For this review, take the finished solid that the model builds, in its own axes (mm). Round coordinates to 2 decimals unless told otherwise and drop trailing zeros. Write each loop counter-clockwise with the first axis right and the second up, starting at its lowest first coordinate (ties: lowest second). Pieces come first, ordered by that corner, then holes. Notation, with made-up numbers: (-36, 29) -> (-4, 29) arc R20 ccw to (-4, 33) -> close; hole circle Ø9 at (74.5, 45). An arc over 180 degrees is marked (long way). Answer as CSV lines item,"result". Start each with the question number.
Item 1: Wall thickness on probe 1 along Z at (x, y) = (25, 4); probe 2 along Y at (x, z) = (10, -4.5); probe 3 along X at (y, z) = (6.5, -1.75): over which ranges is each line inside the solid? List them lowest first. Write a range as from..to.
Item 2: Take a section at A-A on y = 15.5. Give the boundary of the cut face in (x, z), then the cut area to 3 significant figures.
Item 3: Take a section at B-B on z = -3.25. Give the boundary of the cut face in (x, y), then the cut area to 3 significant figures.
Item 4: Take a section at C-C on x = 21. Give the boundary of the cut face in (y, z).
Item 5: For pin 1 Ø1.5 at (y, z) = (13, -1.5) entering from -X; pin 2 Ø1.5 at (y, z) = (16, -3) entering from +X; pin 3 Ø4 at (x, z) = (19, -2.5) entering from -Y, all flat-tipped, find the tip position at first contact; note any pin that passes through.
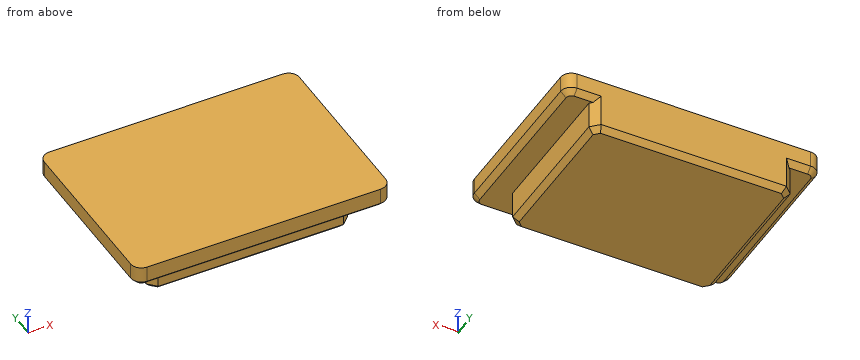
```python
from build123d import *

# Parameters (mm, degrees)
SKETCH1_W           = 37.651513934
SKETCH1_H           = 29.796380505
BOSS_EXTRUDE1_DEPTH = 4
SKETCH1_3_W         = 37.651513934
SKETCH1_3_H         = 29.796380505
BOSS_EXTRUDE2_DEPTH = 6
FILLET1_R           = 2
CHAMFER1_SIZE       = 1.5
CHAMFER2_SIZE       = 1
CHAMFER3_SIZE       = 1


with BuildPart() as part:
    # Sketch1 → Boss-Extrude1 (new body)
    with BuildSketch(Plane.XY):
        Polygon((0, 34.333333333), (0, 0), (47.666666667, 0), (47.666666667, 34.333333333), (42.6590903, 34.333333333), (42.6590903, 4.536952828), (5.007576366, 4.536952828), (5.007576366, 34.333333333), align=None)
        with Locations((23.833333333, 19.43514308)):
            Rectangle(SKETCH1_W, SKETCH1_H)
    extrude(amount=BOSS_EXTRUDE1_DEPTH)

    # Sketch1_3 → Boss-Extrude2 (add)
    with BuildSketch(Plane.XY):
        with Locations((23.833333333, 19.43514308)):
            Rectangle(SKETCH1_3_W, SKETCH1_3_H)
    extrude(amount=-BOSS_EXTRUDE2_DEPTH)

    # Fillet1
    fillet1_edges = [part.edges().sort_by_distance(p)[0] for p in [
        (47.666666667, 34.333333333, 2),
        (47.666666667, 0, 2),
        (0, 0, 2),
        (0, 34.333333333, 2),
    ]]
    fillet(fillet1_edges, radius=FILLET1_R)

    # Chamfer1
    chamfer1_edges = [part.edges().sort_by_distance(p)[0] for p in [
        (42.6590903, 34.333333333, -3),
        (42.6590903, 4.536952828, -3),
        (5.007576366, 4.536952828, -3),
        (5.007576366, 34.333333333, -3),
    ]]
    chamfer(chamfer1_edges, length=CHAMFER1_SIZE)

    # Chamfer2
    chamfer2_edges = [part.edges().sort_by_distance(p)[0] for p in [
        (23.833333333, 34.333333333, -6),
        (5.007576366, 19.435143081, -6),
        (42.6590903, 19.435143081, -6),
        (23.833333333, 4.536952828, -6),
        (5.757576366, 5.286952828, -6),
        (41.9090903, 5.286952828, -6),
        (41.9090903, 33.583333333, -6),
        (5.757576366, 33.583333333, -6),
    ]]
    chamfer(chamfer2_edges, length=CHAMFER2_SIZE)

    # Chamfer3
    chamfer3_edges = [part.edges().sort_by_distance(p)[0] for p in [
        (44.162878483, 34.333333333, 0),
        (0, 17.166666667, 0),
        (47.666666667, 17.166666667, 0),
        (23.833333333, 0, 0),
        (3.503788183, 34.333333333, 0),
        (47.080880229, 0.585786438, 0),
        (0.585786438, 0.585786438, 0),
        (47.080880229, 33.747546896, 0),
        (0.585786438, 33.747546896, 0),
    ]]
    chamfer(chamfer3_edges, length=CHAMFER3_SIZE)


solid = part.part
```
Output values:
1,probe 1,"z = 0..4"
1,probe 2,"y = 4.54..34.33"
1,probe 3,"x = 5.01..42.66"
2,outline,"(0, 1) -> (1, 0) -> (5.01, 0) -> (5.01, -5) -> (6.01, -6) -> (41.66, -6) -> (42.66, -5) -> (42.66, 0) -> (46.67, 0) -> (47.67, 1) -> (47.67, 4) -> (0, 4) -> close"
2,area,"415 mm^2"
3,outline,"(5.01, 6.04) -> (6.51, 4.54) -> (41.16, 4.54) -> (42.66, 6.04) -> (42.66, 32.83) -> (41.16, 34.33) -> (6.51, 34.33) -> (5.01, 32.83) -> close"
3,area,"1,120 mm^2"
4,outline,"(0, 1) -> (1, 0) -> (4.54, 0) -> (4.54, -5) -> (5.54, -6) -> (33.33, -6) -> (34.33, -5) -> (34.33, 4) -> (0, 4) -> close"
5,pin 1,"stops at x = 5.01"
5,pin 2,"stops at x = 42.66"
5,pin 3,"stops at y = 4.54"
